Source: CAD feature listing. Evaluate the final solid. Frame: model axes, mm. Face numbers are marked on the shaded views. A direction names the side the tool comes from. Round coordinates to 2 decimals unless told otherwise and drop trailing zeros. Loops run counter-clockwise (first coordinate to the right, second up) from the corner with the lowest first, then second, coordinate; pieces in that order, holes last. Notation, with made-up numbers: (71, 62) -> (99, 62) arc R10 ccw to (99, 70) -> close; hole circle Ø4 at (-7, -27). An arc over 180 degrees is marked (long way). Return JSON: item names as keys, results as strings. Group by question number.
```python
from build123d import *

# Parameters (mm, degrees)
F1_DEPTH = 19.05
F2_W     = 31.7388475657
F2_H     = 12.6919411123
F3_DEPTH = 50.8
F4_W     = 31.7593351066
F4_H     = 12.702934444
F5_DEPTH = 25.4


with BuildPart() as f1:
    # F0 (on Right) → F1 (new body)
    with BuildSketch(Plane.YZ):
        Polygon((0, 31.7267506936), (0, 0), (44.45, 0), (44.45, 31.7312787083), (31.7450927711, 31.7312787083), (31.7450927711, 19.0298414173), (12.6803467474, 19.0298414173), (12.6803467474, 31.7267506936), align=None)
    extrude(amount=F1_DEPTH)

    # F2 (on face) → F3 (join)
    with BuildSketch(Plane.YZ.offset(19.05)):
        with Locations((28.5805762172, 6.3459705561)):
            Rectangle(F2_W, F2_H)
    extrude(amount=F3_DEPTH)

    # F4 (on face) → F5 (cut)
    with BuildSketch(Plane.XY.offset(12.6919411123)):
        with Locations((53.9703324467, 28.594661504)):
            Rectangle(F4_W, F4_H)
    extrude(amount=-F5_DEPTH, mode=Mode.SUBTRACT)


solid = f1.part
```
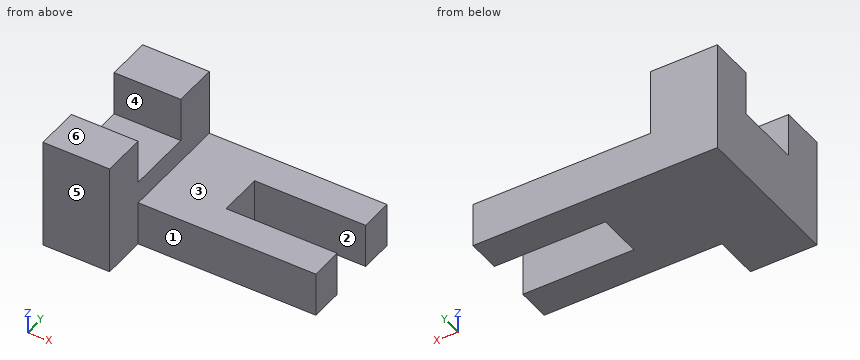
(1) Cut plane A-A (z = 21). Return loops of the section in (x, y).
(2) Cut plane D-D (x = 13). Return loops of the section in (y, z), and give its area (3 significant figures).
(3) Ray query, line 1 (Y direction, x = 66, z = 11.5); line 2 (Z direction, x = 8, y = 5.5); line 3 (Y direction, x = 21, z = 5). Return the intervals inside material, ascending.
(4) Cut plane B-B (x = 43). Return loops of the section in (y, z), and give its area (3 significant figures).
(5) Set-up query: the marked faces 1, 2 and 3. Return all of +Z, -Z, +X, -X, +Y, -Y with unobstructed straight access to the full face (end or side cutting, diameter ignored); none if empty.
(6) Mould query, pull axis Y, two halves, no side actions, for the marked faces 4, 5 and 6. Classes: released by +Y, released by -Y, zero draft, split by the parting line, or undercut.
(7) Cut plane C-C (y = 41). Return loops of the section in (x, z).
(8) Pin query (flat end, axial travel): pin 1 (4 mm diameter, centred on x = 33.5, z = 4, fed in from -Y); pin 2 (1 mm diameter, centred on y = 22.5, z = 16, fed in from +X); pin 3 (15 mm diameter, centred on x = 8, y = 19, fed in from +Z). Return the tip coordinate at first contact, or that it passes through.
Answers follow:
{
 "1": {"outline": "(0, 0) -> (19.05, 0) -> (19.05, 12.68) -> (0, 12.68) -> close; (0, 31.75) -> (19.05, 31.75) -> (19.05, 44.45) -> (0, 44.45) -> close"},
 "2": {"outline": "(0, 0) -> (44.45, 0) -> (44.45, 31.73) -> (31.75, 31.73) -> (31.75, 19.03) -> (12.68, 19.03) -> (12.68, 31.73) -> (0, 31.73) -> close", "area": "1,170 mm^2"},
 "3": {"line 1": "12.71 to 22.24, 34.95 to 44.45", "line 2": "0 to 31.73", "line 3": "12.71 to 44.45"},
 "4": {"outline": "(12.71, 0) -> (22.24, 0) -> (22.24, 12.69) -> (12.71, 12.69) -> close; (34.95, 0) -> (44.45, 0) -> (44.45, 12.69) -> (34.95, 12.69) -> close", "area": "242 mm^2"},
 "5": {"face 1": "+Z, -Z, +X, -Y", "face 2": "+Z, -Z, +X", "face 3": "+Z, +X, +Y, -Y"},
 "6": {"face 4": "undercut", "face 5": "released by -Y", "face 6": "zero draft"},
 "7": {"outline": "(0, 0) -> (69.85, 0) -> (69.85, 12.69) -> (19.05, 12.69) -> (19.05, 31.73) -> (0, 31.73) -> close"},
 "8": {"pin 1": "y = 12.71", "pin 2": "x = 19.05", "pin 3": "z = 31.73"}
}
